For this review, take the finished solid that the model builds, in its own axes (mm). A direction names the side the tool comes from. Give positions to 0.01 mm unless a question says otherwise; leave off trailing zeros. Write each loop counter-clockwise with the first axis right and the second up, starting at its lowest first coordinate (ties: lowest second). Pieces come first, ordered by that corner, then holes. Notation, with made-up numbers: (49, 14.25) -> (77, 14.25) arc R21 cw to (77, 46.25) -> close; hole circle Ø1 at (7, -36.5). An arc over 180 degrees is marked (long way). Return JSON: item names as keys, results as strings.
from build123d import *

# Parameters (mm, degrees)
BOSS_EXTRU_1_DEPTH      = 15
ESQUISSE2_R             = 110
BOSS_EXTRU_2_DEPTH      = 145
ESQUISSE3_R             = 111
ESQUISSE3_R_2           = 108
ENL_V_MAT_EXTRU_1_DEPTH = 4
ESQUISSE4_R             = 5
ENL_V_MAT_EXTRU_2_DEPTH = 471.867329483
CONG_1_R                = 3
CHANFREIN1_SIZE         = 2


with BuildPart() as part:
    # Esquisse1 → Boss.-Extru.1 (new body)
    with BuildSketch(Plane(origin=(0, 0, 0), x_dir=(1, 0, 0), z_dir=(0, 1, 0))):
        with BuildLine():
            Line((-140, 43.338898303), (-140, -43.338898303))
            ThreePointArc((-140, -43.338898303), (-112.630211626, -115.949146387), (-44.140943151, -152.426174036))
            Line((-44.140943151, -152.426174036), (332.286758282, -201.222357555))
            ThreePointArc((332.286758282, -201.222357555), (379.605589864, -186.791231678), (400, -141.720207155))
            Line((400, -141.720207155), (400, 141.720207155))
            ThreePointArc((400, 141.720207155), (379.605589864, 186.791231678), (332.286758282, 201.222357555))
            Line((332.286758282, 201.222357555), (-44.140943151, 152.426174036))
            ThreePointArc((-44.140943151, 152.426174036), (-112.630211626, 115.949146387), (-140, 43.338898303))
        make_face()
    extrude(amount=BOSS_EXTRU_1_DEPTH)

    # Esquisse2 → Boss.-Extru.2 (add)
    with BuildSketch(Plane(origin=(0, 15, 0), x_dir=(1, 0, 0), z_dir=(0, 1, 0))):
        with Locations(Location((0, 0, 0), (0, 0, 270))):
            Circle(ESQUISSE2_R)
    extrude(amount=BOSS_EXTRU_2_DEPTH)

    # Esquisse3 → Enl_v. mat.-Extru.1 (cut)
    with BuildSketch(Plane(origin=(0, 156, 0), x_dir=(1, 0, 0), z_dir=(0, 1, 0))):
        Circle(ESQUISSE3_R)
        with Locations(Location((0, 0, 0), (0, 0, 270))):
            Circle(ESQUISSE3_R_2, mode=Mode.SUBTRACT)
    extrude(amount=-ENL_V_MAT_EXTRU_1_DEPTH, mode=Mode.SUBTRACT)

    # Esquisse4 → Enl_v. mat.-Extru.2 (cut, through all)
    with BuildSketch(Plane(origin=(0, 15, 0), x_dir=(1, 0, 0), z_dir=(0, 1, 0))):
        with Locations(Location((340, -150, 0), (0, 0, 270))):
            Circle(ESQUISSE4_R)
        with Locations(Location((340, 150, 0), (0, 0, 270))):
            Circle(ESQUISSE4_R)
        with Locations(Location((160, -140, 0), (0, 0, 270))):
            Circle(ESQUISSE4_R)
        with Locations(Location((160, 140, 0), (0, 0, 270))):
            Circle(ESQUISSE4_R)
    extrude(amount=-ENL_V_MAT_EXTRU_2_DEPTH, mode=Mode.SUBTRACT)

    # Cong_1
    cong_1_edges = [part.edges().sort_by_distance(p)[0] for p in [
        (0, 15, -110),
    ]]
    fillet(cong_1_edges, radius=CONG_1_R)

    # Chanfrein1
    chanfrein1_edges = [part.edges().sort_by_distance(p)[0] for p in [
        (-112.630211626, 15, 115.949146387),
        (144.072907565, 15, 176.824265796),
        (379.605589864, 15, 186.791231678),
        (400, 15, 0),
        (379.605589864, 15, -186.791231678),
        (144.072907565, 15, -176.824265796),
        (-112.630211626, 15, -115.949146387),
        (-140, 15, 0),
    ]]
    chamfer(chanfrein1_edges, length=CHANFREIN1_SIZE)


solid = part.part
1. For pin 1 (8 mm diameter, centred on y = 93.5, z = 37, fed in from -X); pin 2 (10 mm diameter, centred on x = 212, z = 144, fed in from +Y); pin 3 (4 mm diameter, centred on y = 132.5, z = -8, fed in from -X), all flat-tipped, find the tip position at first contact; note any pin that passes through.
Results found:
{"pin 1": "stops at x = -104.93", "pin 2": "stops at y = 15", "pin 3": "stops at x = -109.84"}
2. Add section A-A, the plane z = 0. State the section outline as (x, y) points, plus the area to 3 significant figures.
Results found:
{"outline": "(-140, 0) -> (400, 0) -> (400, 13) -> (398, 15) -> (113, 15) arc R3 cw to (110, 18) -> (110, 152) -> (108, 152) -> (108, 156) -> (110, 156) -> (110, 160) -> (-110, 160) -> (-110, 156) -> (-108, 156) -> (-108, 152) -> (-110, 152) -> (-110, 18) arc R3 cw to (-113, 15) -> (-138, 15) -> (-140, 13) -> close", "area": "40,000 mm²"}
3. Add section D-D, the plane x = 182.5. State the section outline as (y, z) points.
Results found:
{"outline": "(0, -181.81) -> (13, -181.81) -> (15, -179.79) -> (15, 179.79) -> (13, 181.81) -> (0, 181.81) -> close"}
4. To check wall thickness, follow probe 1 along Z at (x, y) = (340, 4); probe 2 along Y at (x, z) = (106, 155.5); probe 3 along X at (y, z) = (99, 4). State the ranges of each line that lie inside material, in increasing order.
Results found:
{"probe 1": "z = -201.72 to -155, -145 to 145, 155 to 201.72", "probe 2": "y = 0 to 15", "probe 3": "x = -109.93 to 109.93"}
5. For faces 5 (the flat face through (146.835, 13.986, -176.188)), 6 (the flat face through (81, 156, 73)), 7 (the cylindrical face through (-97.59, 157.97, 50.76)), list the 3-axis set-ups (+Z, -Z, +X, -X, +Y, -Y) from which the entire face can be reached by the end or side of a thin tool; tool diameter is ignored.
Results found:
{"face 5": "-Z, -X, +Y", "face 6": "none", "face 7": "+Y"}
6. The part is to be moulded in two halves that separate along Y. For faces 1 (the flat face through (81, 152, 73)), 2 (the flat face through (2, 160, -2)), 3 (the flat face through (400, 6, 2)), 4 (the cylindrical face through (-105.432, 154.028, -23.412)), say which applies: +Y half, -Y half, draft (parallel to the pull), parting line (faces both ways), or undercut.
Results found:
{"face 1": "undercut", "face 2": "+Y half", "face 3": "draft", "face 4": "undercut"}
7. Add section C-C, the plane y = 115. State the section outline as (x, z) points.
Results found:
{"outline": "circle Ø220 at (0, 0)"}
8. Add section B-B, the plane x = 312. State the section outline as (y, z) points, plus the area to 3 significant figures.
Results found:
{"outline": "(0, -198.59) -> (13, -198.59) -> (15, -196.58) -> (15, 196.58) -> (13, 198.59) -> (0, 198.59) -> close", "area": "5,950 mm²"}
